Verification items for the finished model (mm, model axes). A direction names the side the tool comes from. Coordinates: 2 decimals unless noted, no trailing zeros. Loops run counter-clockwise (first coordinate to the right, second up) from the corner with the lowest first, then second, coordinate; pieces in that order, holes last.
Q1. Access from +Z, -Z, +X, -X, +Y, -Y to the whole of each face (thin tool, end or side, straight path). Record for faces 1 (the face through (1.88, -2.26, 12.47)), 2 (the face through (1.878, -6.252, 9.235)), 3 (the face through (2, -17, 8.255)).
Q2. Sectioned sample at A-A (x = 0.9). Enter the section's corners in (y, z) (3 decimals).
Q3. Sectioned sample at C-C (y = -11.5). Enter the section's corners in (x, z) (3 decimals), then the cut area to 3 significant figures.
Q4. Go/stop test with flat-tipped pins: P1, Ø1.1, axis at x = 2.5, y = -17, coming from the -Z side; P2, Ø1.1, axis at x = 2, y = -16, coming from the +Z side (3 decimals). Record where each tip stops, or that it passes through.
Q5. Mould release check, pull along Z, two halves, no side actions. Record for faces 4 (the face through (1.878, -2.542, -6.188)), 5 (the face through (1.878, -1.942, 13.949)), 6 (the face through (1.878, 8.136, -1.398)): +Z half, -Z half, draft (parallel to the pull), parting line (faces both ways), or undercut.
Q6. Material ranges on probe 1 along Z at (x, y) = (1.5, -8.5) (3 decimals); probe 2 along Z at (x, y) = (1.2, 0.5), recorded low to high.
Q7. Sectioned sample at B-B (y = 3). Enter the section's corners in (x, z).
```python
from build123d import *

# Parameters (mm, degrees)
BOSS_EXTRUDE1_DEPTH = 3.81
FILLET1_R           = 2.794


with BuildPart() as part:
    # Sketch1 → Boss-Extrude1 (new body)
    with BuildSketch(Plane(origin=(0, 0, 0), x_dir=(0, 0, -1), z_dir=(1, 0, 0))):
        with BuildLine():
            Line((-5.08, 0), (-5.08, -25.4))
            Line((-5.08, -25.4), (-8.255, -25.4))
            Line((-8.255, -25.4), (-8.255, -2.463960679))
            Line((-8.255, -2.463960679), (-11.554166285, -5.629191448))
            Line((-11.554166285, -5.629191448), (-14.543550901, -2.513312179))
            Line((-14.543550901, -2.513312179), (-13.336585788, -1.355345959))
            Line((-13.336585788, -1.355345959), (-11.57812425, -3.188216118))
            Line((-11.57812425, -3.188216118), (-8.255, 0))
            ThreePointArc((-8.255, 0), (1.598457615, 8.098762761), (7.635965052, -3.136409209))
            Line((7.635965052, -3.136409209), (4.699055417, -1.930097975))
            ThreePointArc((4.699055417, -1.930097975), (0.983666225, 4.983854007), (-5.08, 0))
        make_face()
    extrude(amount=BOSS_EXTRUDE1_DEPTH)

    # Fillet1
    # the kernel refuses this fillet: 2.794 mm, written as the material it adds along each edge
    with BuildSketch(Plane(origin=(0, -2.463960679, 8.255), x_dir=(0, -1, 0), z_dir=(1, 0, 0))) as fillet1_piece_1:
        with BuildLine():
            CenterArc((5.913183284, -2.794), FILLET1_R, 90, 100.416592131)
            Line((3.165230769, -3.299166285), (3.110271719, -3.309269611))
            ThreePointArc((3.110271719, -3.309269611), (1.542292241, -1.688269296), (-0.040323143, -0.038686154))
            Line((-0.040323143, -0.038686154), (0, 0.05588))
            Line((0, 0.05588), (5.913183284, 0.05588))
            Line((5.913183284, 0.05588), (5.913183284, 0))
        make_face()
    extrude(amount=3.81)


solid = part.part
```
Geometry check:
1. face 1: +X, -X, +Y
1. face 2: +X, -X, -Y
1. face 3: +Z, +X, -X, -Y
2. outline: (-25.4, 5.08) - (0, 5.08) arc R5.08 cw (long way) to (-1.93, -4.699) - (-3.136, -7.636) arc R8.255 ccw (long way) to (0, 8.255) - (-3.188, 11.578) - (-1.355, 13.337) - (-2.513, 14.544) - (-5.629, 11.554) arc R2.794 cw to (-8.377, 8.255) - (-25.4, 8.255) - close
3. outline: (0, 5.08) - (3.81, 5.08) - (3.81, 8.255) - (0, 8.255) - close
3. area: 12.1 mm2
4. P1: stops at z = 5.08
4. P2: stops at z = 8.255
5. face 4: undercut
5. face 5: +Z half
5. face 6: parting line
6. probe 1: z = 5.08 to 8.255
6. probe 2: z = -8.24 to -5.06, 5.06 to 8.24
7. outline: (0, -7.69) - (3.81, -7.69) - (3.81, -4.1) - (0, -4.1) - close; (0, 4.1) - (3.81, 4.1) - (3.81, 7.69) - (0, 7.69) - close
